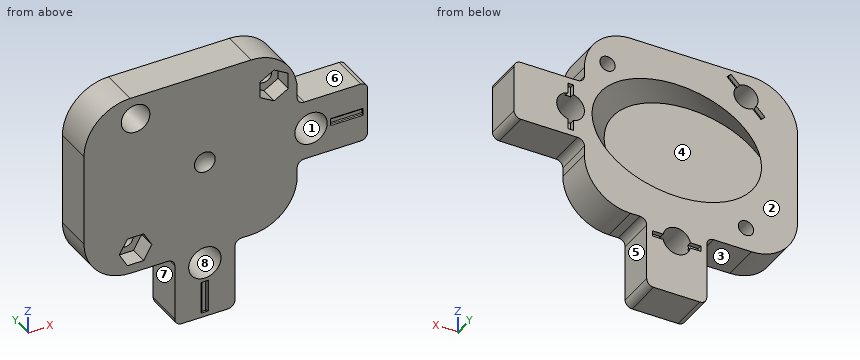
```python
from build123d import *

# Parameters (mm, degrees)
SKETCH2_R           = 3
SKETCH2_R_2         = 2.6
SKETCH2_R_3         = 1.65
BOSS_EXTRUDE1_DEPTH = 8.3
SKETCH19_RX         = 18.35
SKETCH19_RY         = 12.8
CUT_EXTRUDE4_DEPTH  = 8.485281374
FILLET1_R           = 1.5
FILLET2_R           = 10
SKETCH14_W          = 1.2
SKETCH14_H          = 10.4
SKETCH14_W_2        = 10.4
SKETCH14_H_2        = 1.2
CUT_EXTRUDE2_DEPTH  = 1
CUT_EXTRUDE3_DEPTH  = 3.9
CHAMFER1_SIZE       = 0.5
CHAMFER1_SIZE_2     = 8.3
SKETCH20_W          = 7
SKETCH20_H          = 1.2
SKETCH20_W_2        = 1.2
SKETCH20_H_2        = 7
CUT_EXTRUDE5_DEPTH  = 0.4
FILLET3_START       = -35
FILLET3_DEPTH       = 7.75
FILLET3_START_2     = 27.25
FILLET3_2_DEPTH     = 7.75
FILLET3_START_3     = -34.25
FILLET3_3_DEPTH     = 7
FILLET3_4_DEPTH     = 7


with BuildPart() as part:
    # Sketch2 → Boss-Extrude1 (new body)
    with BuildSketch(Plane(origin=(0, 0, 0), x_dir=(1, 0, 0), z_dir=(0, 1, 0))):
        Polygon((20, -20), (20, -6.5), (35.25, -6.5), (35.25, 6.5), (20, 6.5), (20, 20), (6.5, 20), (6.5, 35.25), (-6.5, 35.25), (-6.5, 20), (-26.17, 20), (-26.17, -20), align=None)
        with Locations(Location((23, 0, 0), (0, 0, 90))):
            Circle(SKETCH2_R, mode=Mode.SUBTRACT)
        with Locations(Location((0, 23, 0), (0, 0, 90))):
            Circle(SKETCH2_R, mode=Mode.SUBTRACT)
        with Locations(Location((-15, -15, 0), (0, 0, 90))):
            Circle(SKETCH2_R_2, mode=Mode.SUBTRACT)
        with Locations(Location((-15, 15, 0), (0, 0, 90))):
            Circle(SKETCH2_R_3, mode=Mode.SUBTRACT)
        with Locations(Location((15, -12.5, 0), (0, 0, 90))):
            Circle(SKETCH2_R_3, mode=Mode.SUBTRACT)
    extrude(amount=BOSS_EXTRUDE1_DEPTH)

    # Sketch19 → Cut-Extrude4 (cut, along a direction that is not the sketch's normal)
    with BuildSketch(Plane(origin=(11.72685066, 8.3, 0), x_dir=(0, 0, -1), z_dir=(0, 1, 0))):
        with Locations(Location((0, 11.72685066), (0, 0, 90))):
            Ellipse(SKETCH19_RX, SKETCH19_RY)
    extrude(amount=-CUT_EXTRUDE4_DEPTH, dir=(0.7071067811865488, 0.7071067811865464, 0), mode=Mode.SUBTRACT)

    # Fillet1
    fillet1_edges = [part.edges().sort_by_distance(p)[0] for p in [
        (-6.5, 4.15, -20),
        (-6.5, 4.15, -35.25),
        (6.5, 4.15, -35.25),
        (6.5, 4.15, -20),
        (20, 4.15, -6.5),
        (35.25, 4.15, -6.5),
        (35.25, 4.15, 6.5),
        (20, 4.15, 6.5),
    ]]
    fillet(fillet1_edges, radius=FILLET1_R)

    # Fillet2
    fillet2_edges = [part.edges().sort_by_distance(p)[0] for p in [
        (-26.17, 4.15, 20),
        (-26.17, 4.15, -20),
        (20, 4.15, -20),
        (20, 4.15, 20),
    ]]
    fillet(fillet2_edges, radius=FILLET2_R)

    # Sketch15 → Cut-Revolve1 (revolve, cut)
    with BuildSketch(Plane.XY):
        with BuildLine():
            Line((0, 0), (0, 1.2))
            ThreePointArc((0, 1.2), (1.272792206, 0.88117618), (2.244994432, 0))
            Line((2.244994432, 0), (0, 0))
        make_face()
    revolve(axis=Axis((0, 0, 0), (0, 1, 0)), mode=Mode.SUBTRACT)

    # Sketch14 → Cut-Extrude2 (cut)
    with BuildSketch(Plane(origin=(0, 8.3, 0), x_dir=(1, 0, 0), z_dir=(0, 1, 0))):
        with Locations((23, 0)):
            Rectangle(SKETCH14_W, SKETCH14_H)
        with Locations((0, 23)):
            Rectangle(SKETCH14_W_2, SKETCH14_H_2)
        Polygon((-18.252691193, -10.898780669), (-10.898780669, -18.252691193), (-11.747308807, -19.101219331), (-19.101219331, -11.747308807), align=None)
    extrude(amount=-CUT_EXTRUDE2_DEPTH, mode=Mode.SUBTRACT)

    # Sketch16 → Cut-Extrude3 (cut)
    with BuildSketch(Plane.XZ):
        Polygon((-13.239081679, -11.95), (-16.760918321, -11.95), (-18.521836642, -15), (-16.760918321, -18.05), (-13.239081679, -18.05), (-11.478163358, -15), align=None)
        Polygon((18.05, 14.260918321), (15, 16.021836642), (11.95, 14.260918321), (11.95, 10.739081679), (15, 8.978163358), (18.05, 10.739081679), align=None)
    extrude(amount=-CUT_EXTRUDE3_DEPTH, mode=Mode.SUBTRACT)

    # Chamfer1
    # the kernel refuses this chamfer: 8.3, 0.5 mm, written as the material it takes off along each edge
    with BuildSketch(Plane(origin=(0, 0, -23), x_dir=(0, 0, -1), z_dir=(1, 0, 0))) as chamfer1_piece_1:
        Polygon((3 + CHAMFER1_SIZE, 0), (3, CHAMFER1_SIZE_2), (3, 0), align=None)
    revolve(axis=Axis((0, 0, -23), (0, 1, 0)), mode=Mode.SUBTRACT)
    with BuildSketch(Plane(origin=(23, 0, 0), x_dir=(0, 0, -1), z_dir=(1, 0, 0))) as chamfer1_piece_2:
        Polygon((3 + CHAMFER1_SIZE, 0), (3, CHAMFER1_SIZE_2), (3, 0), align=None)
    revolve(axis=Axis((23, 0, 0), (0, 1, 0)), mode=Mode.SUBTRACT)
    with BuildSketch(Plane(origin=(-15, 0, 15), x_dir=(0, 0, -1), z_dir=(1, 0, 0))) as chamfer1_piece_3:
        Polygon((2.6 + CHAMFER1_SIZE, 0), (2.6, CHAMFER1_SIZE_2), (2.6, 0), align=None)
    revolve(axis=Axis((-15, 0, 15), (0, 1, 0)), mode=Mode.SUBTRACT)

    # Sketch20 → Cut-Extrude5 (cut)
    with BuildSketch(Plane.XZ):
        with Locations((30.75, 0)):
            Rectangle(SKETCH20_W, SKETCH20_H)
        with Locations((0, -30.75)):
            Rectangle(SKETCH20_W_2, SKETCH20_H_2)
    extrude(amount=-CUT_EXTRUDE5_DEPTH, mode=Mode.SUBTRACT)

    # Fillet3: read off the stored shape, not the designer's step
    # Fillet3 outline → Fillet3 (add)
    with BuildSketch(Plane.XY.offset(FILLET3_START)):
        with BuildLine():
            ThreePointArc((-0.6, 0.2), (-0.541421356, 0.341421356), (-0.4, 0.4))
            Line((-0.4, 0.4), (-0.6, 0.4))
            Line((-0.6, 0.4), (-0.6, 0.2))
        make_face()
        with BuildLine():
            Line((0.6, 0.4), (0.4, 0.4))
            ThreePointArc((0.4, 0.4), (0.541421356, 0.341421356), (0.6, 0.2))
            Line((0.6, 0.2), (0.6, 0.4))
        make_face()
    extrude(amount=FILLET3_DEPTH)

    # Fillet3 2 outline → Fillet3 2 (add)
    with BuildSketch(Plane.YZ.offset(FILLET3_START_2)):
        with BuildLine():
            Line((0.4, -0.6), (0.4, -0.4))
            ThreePointArc((0.4, -0.4), (0.341421356, -0.541421356), (0.2, -0.6))
            Line((0.2, -0.6), (0.4, -0.6))
        make_face()
        with BuildLine():
            ThreePointArc((0.2, 0.6), (0.341421356, 0.541421356), (0.4, 0.4))
            Line((0.4, 0.4), (0.4, 0.6))
            Line((0.4, 0.6), (0.2, 0.6))
        make_face()
    extrude(amount=FILLET3_2_DEPTH)

    # Fillet3 3 outline → Fillet3 3 (cut)
    with BuildSketch(Plane.XY.offset(FILLET3_START_3)):
        with BuildLine():
            Line((-0.6, 0), (-0.6, 0.2))
            ThreePointArc((-0.6, 0.2), (-0.658578644, 0.058578644), (-0.8, 0))
            Line((-0.8, 0), (-0.6, 0))
        make_face()
        with BuildLine():
            ThreePointArc((0.8, 0), (0.658578644, 0.058578644), (0.6, 0.2))
            Line((0.6, 0.2), (0.6, 0))
            Line((0.6, 0), (0.8, 0))
        make_face()
    extrude(amount=FILLET3_3_DEPTH, mode=Mode.SUBTRACT)

    # Fillet3 4 outline → Fillet3 4 (cut)
    with BuildSketch(Plane.YZ.offset(FILLET3_START_2)):
        with BuildLine():
            ThreePointArc((0, -0.8), (0.058578644, -0.658578644), (0.2, -0.6))
            Line((0.2, -0.6), (0, -0.6))
            Line((0, -0.6), (0, -0.8))
        make_face()
        with BuildLine():
            Line((0, 0.6), (0.2, 0.6))
            ThreePointArc((0.2, 0.6), (0.058578644, 0.658578644), (0, 0.8))
            Line((0, 0.8), (0, 0.6))
        make_face()
    extrude(amount=FILLET3_4_DEPTH, mode=Mode.SUBTRACT)


solid = part.part
```
Part model, mm, in its own coordinate system. Face numbers are marked on the shaded views. A direction names the side the tool comes from. Round coordinates to 2 decimals unless told otherwise and drop trailing zeros. Write each loop counter-clockwise with the first axis right and the second up, starting at its lowest first coordinate (ties: lowest second). Pieces come first, ordered by that corner, then holes. Notation, with made-up numbers: M -15.5,-7.5 L 38.5,-7.5 A5 cw 38.5,-3.5 Z; hole C 56,-23.75 d2. An arc over 180 degrees is marked long. Answer as CSV lines item,"result". Start each with the question number.
1) Mould opens along Z. For the marked faces 1, 2 and 3 say: +Z half, -Z half, draft (parallel to the pull), parting line (faces both ways), or undercut.
2) Band-saw the part on A-A (z = 15). List the corners of the cut face in (x, y).
3) Drill centre lines: L1, parallel to Z at x = -15, y = 6; L2, parallel to Z at x = -15, y = 6.5; L3, parallel to X at y = 7.5, z = 13. Where is each one in solid material? Low to high.
4) Which spindle directions (+Z, -Z, +X, -X, +Y, -Y) get a long thin tool onto all of the face, cutting with end or side? Do the marked faces 4, 5, 6, 7 and 8. Say none if no direction does.
5) Drop flat-ended pins along their axis: pin 1 (5 mm diameter, centred on x = 10.5, z = -2.5, fed in from -Y); pin 2 (1.8 mm diameter, centred on x = 15, z = 14, fed in from -Y); pin 3 (2.5 mm diameter, centred on x = 27, y = 2.5, fed in from -Z); pin 4 (8 mm diameter, centred on x = 14, z = -29, fed in from -Y). Give the stop position or say it passes through.
Worked out:
1,face 1,"undercut"
1,face 2,"draft"
1,face 3,"-Z half"
2,outline,"M -24.83,0 L -18.1,0 L -17.6,8.3 L -24.83,8.3 Z; M -12.4,8.3 L -11.9,0 L 13.23,0 L 13.23,3.9 L 16.77,3.9 L 16.77,0 L 18.66,0 L 18.66,8.3 Z"
3,L1,"-20 to -16.65, -13.35 to -9.24, 9.24 to 12.26, 17.74 to 20"
3,L2,"-20 to -16.65, -13.35 to -8.89, 8.89 to 12.29, 17.71 to 20"
3,L3,"-25.71 to -17.85, -13.26 to 13.43, 16.57 to 19.54"
4,face 4,"none"
4,face 5,"-Z, +X, +Y, -Y"
4,face 6,"+Z, +X, +Y, -Y"
4,face 7,"-Z, -X, +Y, -Y"
4,face 8,"-Y"
5,pin 1,"y = 0"
5,pin 2,"y = 3.9"
5,pin 3,"z = -6.5"
5,pin 4,"through"
